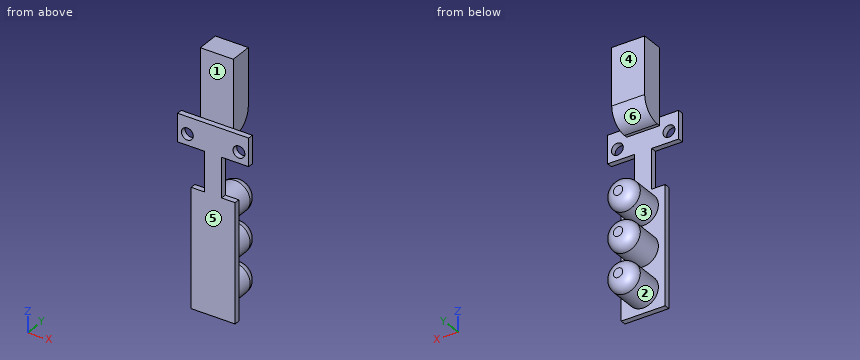
from build123d import *

# Parameters (mm, degrees)
SKETCH1_W           = 13.208
SKETCH1_H           = 35.56
SKETCH1_W_2         = 5.08
SKETCH1_H_2         = 11.938
SKETCH1_W_3         = 21.336
SKETCH1_H_3         = 8.382
SKETCH1_R           = 1.778
BOSS_EXTRUDE1_DEPTH = 1.651
SKETCH2_R           = 4.572
BOSS_EXTRUDE2_DEPTH = 11.303
FILLET1_R           = 3.175
SKETCH3_W           = 9.906
SKETCH3_H           = 2.54
SKETCH3_H_2         = 20.32
BOSS_EXTRUDE3_DEPTH = 6.731
FILLET2_R           = 5.715


with BuildPart() as part:
    # Sketch1 → Boss-Extrude1 (new body)
    # profile 1 of 3: a face of its own
    with BuildSketch(Plane(origin=(0, 0, 0), x_dir=(1, 0, 0), z_dir=(0, 1, 0))):
        Rectangle(SKETCH1_W, SKETCH1_H)
    # profile 2 of 3: a face of its own
    with BuildSketch(Plane(origin=(0, 0, 0), x_dir=(1, 0, 0), z_dir=(0, 1, 0))):
        with Locations((0, -23.749)):
            Rectangle(SKETCH1_W_2, SKETCH1_H_2)
    # profile 3 of 3: a face of its own
    with BuildSketch(Plane(origin=(0, 0, 0), x_dir=(1, 0, 0), z_dir=(0, 1, 0))):
        with Locations((0, -33.909)):
            Rectangle(SKETCH1_W_3, SKETCH1_H_3)
        with Locations(Location((-7.747, -33.02, 0), (0, 0, 90))):
            Circle(SKETCH1_R, mode=Mode.SUBTRACT)
        with Locations(Location((7.747, -33.02, 0), (0, 0, 90))):
            Circle(SKETCH1_R, mode=Mode.SUBTRACT)
    extrude(amount=BOSS_EXTRUDE1_DEPTH)

    # Sketch2 → Boss-Extrude2 (add)
    with BuildSketch(Plane(origin=(0, 1.651, 0), x_dir=(1, 0, 0), z_dir=(0, 1, 0))):
        with Locations(Location((0, 11.6205, 0), (0, 0, 90))):
            Circle(SKETCH2_R)
        with Locations(Location((0, -0.4445, 0), (0, 0, 90))):
            Circle(SKETCH2_R)
        with Locations(Location((0, -12.5095, 0), (0, 0, 90))):
            Circle(SKETCH2_R)
    extrude(amount=BOSS_EXTRUDE2_DEPTH)

    # Fillet1
    fillet1_edges = [part.edges().sort_by_distance(p)[0] for p in [
        (0, 12.954, -7.0485),
        (0, 12.954, 5.0165),
        (0, 12.954, 17.0815),
    ]]
    fillet(fillet1_edges, radius=FILLET1_R)

    # Sketch3 → Boss-Extrude3 (add)
    with BuildSketch(Plane(origin=(0, 1.651, 0), x_dir=(1, 0, 0), z_dir=(0, 1, 0))):
        with Locations((0, -36.83)):
            Rectangle(SKETCH3_W, SKETCH3_H)
        with Locations((0, -48.26)):
            Rectangle(SKETCH3_W, SKETCH3_H_2)
    extrude(amount=BOSS_EXTRUDE3_DEPTH)

    # Fillet2
    fillet2_edges = [part.edges().sort_by_distance(p)[0] for p in [
        (0, 8.382, 35.56),
    ]]
    fillet(fillet2_edges, radius=FILLET2_R)


solid = part.part
Read the model definition and answer for the solid it produces. Units are mm, in the model's axes. Face numbers are marked on the shaded views. A direction names the side the tool comes from. Round coordinates to 2 decimals unless told otherwise and drop trailing zeros. Order: outer loops, then holes, each group sorted by start corner. A loop starts at its lowest first (then second) coordinate and runs counter-clockwise, first axis right, second up.
1) Straight lines are drawn through the part: L1, parallel to X at y = 0.75, z = 33.02 (3 decimals); L2, parallel to Z at x = 1, y = 9.5; L3, parallel to Z at x = -1.25, y = 10. For each, find the intervals that lie inside material, in ascending order.
2) The part is cut by section A-A on z = 33.02. Write down the section's boundary in (x, y) (3 decimals), plus the area to 3 significant figures.
3) The part is cut by section B-B on y = 6.5. Write down the section's boundary in (x, z).
4) The part is cut by section D-D on y = 12. Give the number of separate pieces and of enclosed holes in the cut face, plus the area to 3 significant figures.
5) Flat-ended cylindrical pins translate along their axes: pin 1 (0.5 mm diameter, centred on y = 1, z = -6, fed in from +X); pin 2 (11 mm diameter, centred on x = -2, z = 49, fed in from -Y); pin 3 (3 mm diameter, centred on x = 3, y = 9.5, fed in from +Z); pin 4 (0.5 mm diameter, centred on x = 4, y = 1, fed in from +Z). Find the tip coordinate at first contact, or state that the pin passes through.
6) The part is cut by section C-C on z = 50. Write down the section's boundary in (x, y).
7) The mould has two halves that part along Z. Classify the marked faces 1 and 2: released by +Z, released by -Z, zero draft, split by the parting line, or undercut.
8) For the marked faces 3, 4, 5 and 6, determine the directions among +Z, -Z, +X, -X, +Y, -Y from which every point of the face is accessible in a straight line to the end or side of a thin tool.
Resolved:
1. L1: x = -10.668 to -9.525, -5.969 to 5.969, 9.525 to 10.668
1. L2: z = -16.08 to -7.16, -4.02 to 4.91, 8.05 to 16.97
1. L3: z = -16.01 to -7.23, -3.95 to 4.83, 8.12 to 16.9
2. outline: (-10.668, 0) - (-9.525, 0) - (-9.525, 1.651) - (-10.668, 1.651) - close; (-5.969, 0) - (5.969, 0) - (5.969, 1.651) - (-5.969, 1.651) - close; (9.525, 0) - (10.668, 0) - (10.668, 1.651) - (9.525, 1.651) - close
2. area: 23.5 mm2
3. outline: (-4.95, 37.04) - (4.95, 37.04) - (4.95, 58.42) - (-4.95, 58.42) - close; circle Ø9.14 at (0, -11.62); circle Ø9.14 at (0, 0.44); circle Ø9.14 at (0, 12.51)
4. separate pieces: 3
4. enclosed holes: 0
4. area: 127 mm2
5. pin 1: stops at x = 6.6
5. pin 2: stops at y = 1.65
5. pin 3: stops at z = 58.42
5. pin 4: stops at z = 38.1
6. outline: (-4.95, 1.65) - (4.95, 1.65) - (4.95, 8.38) - (-4.95, 8.38) - close
7. face 1: zero draft
7. face 2: undercut
8. face 3: +Y
8. face 4: +Z, +X, -X, +Y
8. face 5: +Z, -Z, +X, -X, -Y
8. face 6: +X, -X, +Y
